```python
from build123d import *

# Parameters (mm, degrees)
F0_W     = 660.4
F0_H     = 76.2
F1_DEPTH = 38.1
F2_W     = 660.4
F2_H     = 66.675
F3_DEPTH = 33.3375
F5_DEPTH = 25.4


with BuildPart() as f1:
    # F0 (on Front) → F1 (new body)
    with BuildSketch(Plane.XZ):
        with Locations((-11.768971, -10.047171)):
            Rectangle(F0_W, F0_H)
    extrude(amount=-F1_DEPTH)

    # F2 (on face) → F3 (cut)
    with BuildSketch(Plane.XZ):
        with Locations((-11.768971, -10.047171)):
            Rectangle(F2_W, F2_H)
    extrude(amount=-F3_DEPTH, mode=Mode.SUBTRACT)

    # F4 (on face) → F5 (cut)
    with BuildSketch(Plane.XZ.offset(-33.3375)):
        Polygon((-277.675221, 7.514036), (-283.231471, -2.109671), (-277.675221, -11.733378), (-266.562721, -11.733378), (-261.006471, -2.109671), (-266.562721, 7.514036), align=None)
        Polygon((-150.675221, 7.514036), (-156.231471, -2.109671), (-150.675221, -11.733378), (-139.562721, -11.733378), (-134.006471, -2.109671), (-139.562721, 7.514036), align=None)
        Polygon((-23.675221, 7.514036), (-29.231471, -2.109671), (-23.675221, -11.733378), (-12.562721, -11.733378), (-7.006471, -2.109671), (-12.562721, 7.514036), align=None)
        Polygon((103.324779, 7.514036), (97.768529, -2.109671), (103.324779, -11.733378), (114.437279, -11.733378), (119.993529, -2.109671), (114.437279, 7.514036), align=None)
        Polygon((230.324779, 7.514036), (224.768529, -2.109671), (230.324779, -11.733378), (241.437279, -11.733378), (246.993529, -2.109671), (241.437279, 7.514036), align=None)
    extrude(amount=-F5_DEPTH, mode=Mode.SUBTRACT)


solid = f1.part
```
Could you check a few things on this model? Use its own coordinates, in mm. A direction names the side the tool comes from. Round coordinates to 2 decimals unless told otherwise and drop trailing zeros. Loops run counter-clockwise (first coordinate to the right, second up) from the corner with the lowest first, then second, coordinate; pieces in that order, holes last. Notation, with made-up numbers: (52, 85) -> (105, 85) arc R35 ccw to (105, 117) -> close; hole circle Ø9 at (78.5, 58). An arc over 180 degrees is marked (long way). Put each result on its own line as item: value.
Q1. I want a section at C-C on z = -38. Write out the boundary of the cut face in (x, y).
Checks:
outline: (-341.97, 33.34) -> (318.43, 33.34) -> (318.43, 38.1) -> (-341.97, 38.1) -> close
Q2. Thinking about a two-plate mould opening in Z: for faces 3 (the flat face through (-16, 19, 28.053)), 4 (the flat face through (-16, 16, 23.29)), 5 (the flat face through (-16, 38.1, -18)), which applies, pulls with the +Z half, pulls with the -Z half, needs draft (parallel to the pull), parting line crosses it, or undercut?
Checks:
face 3: pulls with the +Z half
face 4: undercut
face 5: needs draft
Q3. I want a section at A-A on y = 11.5. Write out the boundary of the cut face in (x, z), and give its area (3 significant figures).
Checks:
outline: (-341.97, -48.15) -> (318.43, -48.15) -> (318.43, -43.38) -> (-341.97, -43.38) -> close; (-341.97, 23.29) -> (318.43, 23.29) -> (318.43, 28.05) -> (-341.97, 28.05) -> close
area: 6,290 mm2
Q4. Which directions (+Z, -Z, +X, -X, +Y, -Y) give clear straight access to the entire face, cutting with the end or side of a thin tool? Please do faces 1 (the flat face through (-16, 19, -48.147)), 2 (the flat face through (-16, 16, -43.385)).
Checks:
face 1: -Z, +X, -X, +Y, -Y
face 2: +X, -X, -Y
Q5. Please list where these lines run through material, in increasing order: line 1 (Z direction, x = 286.5, y = 23.5); line 2 (Y direction, x = 283.5, z = -17); line 3 (Z direction, x = -263, y = 35.5). Write a range as from..to.
Checks:
line 1: -48.15..-43.38, 23.29..28.05
line 2: 33.34..38.1
line 3: -48.15..-5.56, 1.34..28.05
Q6. I want a section at B-B on x = -181. Write out the boundary of the cut face in (y, z), and give its area (3 significant figures).
Checks:
outline: (0, -48.15) -> (38.1, -48.15) -> (38.1, 28.05) -> (0, 28.05) -> (0, 23.29) -> (33.34, 23.29) -> (33.34, -43.38) -> (0, -43.38) -> close
area: 680 mm2
